Geometry: final body of the model. Coordinates: model frame, mm. A direction names the side the tool comes from. Coordinates: 2 decimals unless noted, no trailing zeros. Order: outer loops, then holes, each group sorted by start corner. A loop starts at its lowest first (then second) coordinate and runs counter-clockwise, first axis right, second up. Notation, with made-up numbers: (81, 46.25) -> (105, 46.25) arc R24 ccw to (105, 83.25) -> close; hole circle Ø9 at (89.5, 74). An arc over 180 degrees is marked (long way). Answer in a Markdown table with one row per item. Add a question column.
1) Section query A-A on y = 0. Return the cut outline in (x, z).
2) Section query C-C on y = 28. Return the cut outline in (x, z), then the cut area to 3 significant figures.
3) Pull-direction query (Y, two-part tool) for faces 1 (the face through (40, 50.8, -1)), 2 (the face through (40, -50.8, -1)), 3 (the face through (40, -1, 50.8)), 4 (the face through (3.736, -18.163, 49.858)); classes: +Y half, -Y half, draft (parallel to the pull), parting line (faces both ways), or undercut.
4) Section query B-B on x = 69. Return the cut outline in (y, z).
5) Contact query for flat-ended pins moving along their axis: P1, Ø10, axis at y = 39, z = -19.5, coming from the +X side; P2, Ø0.5, axis at x = 15, z = 50.5, coming from the -Y side; P3, Ø1.7, axis at y = 4, z = 50, coming from the -X side. Output: stop coordinate, or through.
6) Set-up query: faces 5 (the face through (3.736, 18.163, 49.858)), 6 (the face through (40.915, 47.827, -47.748)), 7 (the face through (0.95, 0.64, 48.68)). Return all of +Z, -Z, +X, -X, +Y, -Y with unobstructed straight access to the full face (end or side cutting, diameter ignored); none if empty.
7) Section query D-D on z = -5. Return the cut outline in (x, y).
8) Ray query, line 1 (Y direction, x = 37, z = -44.5); line 2 (Z direction, x = 39, y = -30); line 3 (X direction, y = -6.5, z = -31). Return the intervals inside material, ascending. Write a range as from..to.
```python
from build123d import *

# Parameters (mm, degrees)
F0_W          = 101.6
F0_H          = 101.6
F0_W_2        = 98.552
F0_H_2        = 98.552
F1_DEPTH      = 76.2
F2_W          = 101.6
F2_H          = 101.6
F3_DEPTH      = 1.524
F4_W          = 38.1
F4_H          = 38.1
F5_DEPTH      = 1.524
F6_R          = 5.08
F7_R          = 5.08
F10_T1_DEPTH  = 93.472
F10_T3_DEPTH  = 88.392
F10_T5_DEPTH  = 74.676
F10_T7_DEPTH  = 69.596
F10_S11_W     = 5.08
F10_S11_H     = 5.08
F10_T12_DEPTH = 5.08
F10_S17_W     = 5.08
F10_S17_H     = 5.08
F10_T18_DEPTH = 5.08
F10_T21_DEPTH = 91.44
F10_T23_DEPTH = 91.44
F10_T26_ANGLE = 90
F10_T28_ANGLE = 90
F10_T30_ANGLE = 90
F10_T32_ANGLE = 90


# Not quite as in the source:
# - a fillet or chamfer that OpenCascade refuses, or shapes differently, is made with other operations: its cross-section is extruded or revolved along the edge and cut away or added
# - a feature of the source that left no trace in its solid (it failed there, or was rolled back) is left out


with BuildPart() as f1:
    # F0 (on Right) → F1 (new body)
    with BuildSketch(Plane.YZ):
        Rectangle(F0_W, F0_H)
        Rectangle(F0_W_2, F0_H_2, mode=Mode.SUBTRACT)
    extrude(amount=F1_DEPTH)

    # F2 (on Right) → F3 (join)
    with BuildSketch(Plane.YZ):
        Rectangle(F2_W, F2_H)
    extrude(amount=F3_DEPTH)

    # F4 (on face) → F5 (cut)
    with BuildSketch(Plane.XY.offset(50.8)):
        with Locations((20.574, 0)):
            Rectangle(F4_W, F4_H)
    extrude(amount=-F5_DEPTH, mode=Mode.SUBTRACT)

    # F6
    f6_edges = [f1.edges().sort_by_distance(p)[0] for p in [
        (39.624, 19.05, 50.038),
        (39.624, -19.05, 50.038),
        (1.524, -19.05, 50.038),
        (1.524, 19.05, 50.038),
    ]]
    fillet(f6_edges, radius=F6_R)

    # F7
    f7_edges = [f1.edges().sort_by_distance(p)[0] for p in [
        (38.1, 50.8, 50.8),
        (38.1, -50.8, 50.8),
        (38.1, -50.8, -50.8),
        (38.1, 50.8, -50.8),
    ]]
    fillet(f7_edges, radius=F7_R)

    # F10: fillet of radius 5.08 on 15 edges, made by hand

    # F10_s2 → F10_t1 (join)
    with BuildSketch(Plane.XY.offset(-44.196)):
        with BuildLine():
            ThreePointArc((1.524, 44.196), (3.0118975516, 47.7881024484), (6.604, 49.276))
            Line((6.604, 49.276), (1.524, 49.276))
            Line((1.524, 49.276), (1.524, 44.196))
        make_face()
        with BuildLine():
            ThreePointArc((1.524, -44.196), (3.0118975516, -47.7881024484), (6.604, -49.276))
            Line((6.604, -49.276), (1.524, -49.276))
            Line((1.524, -49.276), (1.524, -44.196))
        make_face()
    extrude(amount=F10_T1_DEPTH)

    # F10_s4 → F10_t3 (join)
    with BuildSketch(Plane.XZ.offset(-44.196)):
        with BuildLine():
            ThreePointArc((1.524, -44.196), (3.0118975516, -47.7881024484), (6.604, -49.276))
            Line((6.604, -49.276), (1.524, -49.276))
            Line((1.524, -49.276), (1.524, -44.196))
        make_face()
    extrude(amount=F10_T3_DEPTH)

    # F10_s6 → F10_t5 (join)
    with BuildSketch(Plane.YZ.offset(1.524)):
        with BuildLine():
            ThreePointArc((-49.276, 44.196), (-47.7881024484, 47.7881024484), (-44.196, 49.276))
            Line((-44.196, 49.276), (-49.276, 49.276))
            Line((-49.276, 49.276), (-49.276, 44.196))
        make_face()
        with BuildLine():
            ThreePointArc((44.196, 49.276), (47.7881024484, 47.7881024484), (49.276, 44.196))
            Line((49.276, 44.196), (49.276, 49.276))
            Line((49.276, 49.276), (44.196, 49.276))
        make_face()
    extrude(amount=F10_T5_DEPTH)

    # F10_s8 → F10_t7 (join)
    with BuildSketch(Plane.YZ.offset(6.604)):
        with BuildLine():
            ThreePointArc((-49.276, -44.196), (-47.7881024484, -47.7881024484), (-44.196, -49.276))
            Line((-44.196, -49.276), (-49.276, -49.276))
            Line((-49.276, -49.276), (-49.276, -44.196))
        make_face()
        with BuildLine():
            ThreePointArc((49.276, -44.196), (47.7881024484, -47.7881024484), (44.196, -49.276))
            Line((44.196, -49.276), (49.276, -49.276))
            Line((49.276, -49.276), (49.276, -44.196))
        make_face()
    extrude(amount=F10_T7_DEPTH)


with BuildPart() as f10_tool10:
    # F10_s11 → F10_t12 (new body)
    with BuildSketch(Plane.XY.offset(-44.196)):
        with Locations((4.064, 46.736)):
            Rectangle(F10_S11_W, F10_S11_H)
    extrude(amount=-F10_T12_DEPTH)

    # F10_s13 → F10_t14 (revolve, cut)
    with BuildSketch(Plane(origin=(6.604, 44.196, -44.196), x_dir=(0.7071067812, -0.7071067812, 0), z_dir=(0.7071067812, 0.7071067812, 0))):
        with BuildLine():
            ThreePointArc((0, -5.08), (5.08, 0), (0, 5.08))
            Line((0, 5.08), (0, -5.08))
        make_face()
    revolve(axis=Axis((6.604, 44.196, -44.196), (0, 0, -1)), mode=Mode.SUBTRACT)


with BuildPart() as f1_1:
    add(f1.part)

    # F10_t9: union F10_tool10
    add(f10_tool10.part)


with BuildPart() as f10_tool16:
    # F10_s17 → F10_t18 (new body)
    with BuildSketch(Plane.XY.offset(-44.196)):
        with Locations((4.064, -46.736)):
            Rectangle(F10_S17_W, F10_S17_H)
    extrude(amount=-F10_T18_DEPTH)

    # F10_s19 → F10_t20 (revolve, cut)
    with BuildSketch(Plane(origin=(6.604, -44.196, -44.196), x_dir=(0.7071067812, 0.7071067812, 0), z_dir=(-0.7071067812, 0.7071067812, 0))):
        with BuildLine():
            ThreePointArc((0, -5.08), (5.08, 0), (0, 5.08))
            Line((0, 5.08), (0, -5.08))
        make_face()
    revolve(axis=Axis((6.604, -44.196, -44.196), (0, 0, -1)), mode=Mode.SUBTRACT)


with BuildPart() as f1_2:
    add(f1_1.part)

    # F10_t15: union F10_tool16
    add(f10_tool16.part)

    # F10_s22 → F10_t21 (cut)
    with BuildSketch(Plane.XZ.offset(-45.72)):
        with BuildLine():
            ThreePointArc((5.08, 50.8), (1.4878975516, 49.3121024484), (0, 45.72))
            Line((0, 45.72), (0, 50.8))
            Line((0, 50.8), (5.08, 50.8))
        make_face()
        with BuildLine():
            ThreePointArc((5.08, -50.8), (1.4878975516, -49.3121024484), (0, -45.72))
            Line((0, -45.72), (0, -50.8))
            Line((0, -50.8), (5.08, -50.8))
        make_face()
    extrude(amount=F10_T21_DEPTH, mode=Mode.SUBTRACT)

    # F10_s24 → F10_t23 (cut)
    with BuildSketch(Plane.XY.offset(-45.72)):
        with BuildLine():
            ThreePointArc((5.08, 50.8), (1.4878975516, 49.3121024484), (0, 45.72))
            Line((0, 45.72), (0, 50.8))
            Line((0, 50.8), (5.08, 50.8))
        make_face()
        with BuildLine():
            ThreePointArc((5.08, -50.8), (1.4878975516, -49.3121024484), (0, -45.72))
            Line((0, -45.72), (0, -50.8))
            Line((0, -50.8), (5.08, -50.8))
        make_face()
    extrude(amount=F10_T23_DEPTH, mode=Mode.SUBTRACT)

    # F10_s25 → F10_t26 (revolve, cut)
    with BuildSketch(Plane.XY.offset(-45.72)):
        with BuildLine():
            ThreePointArc((5.08, 50.8), (1.4878975516, 49.3121024484), (0, 45.72))
            Line((0, 45.72), (0, 50.8))
            Line((0, 50.8), (5.08, 50.8))
        make_face()
    revolve(axis=Axis((0, 45.72, -45.72), (-1, 0, 0)), revolution_arc=F10_T26_ANGLE, mode=Mode.SUBTRACT)

    # F10_s27 → F10_t28 (revolve, cut)
    with BuildSketch(Plane.XZ.offset(-45.72)):
        with BuildLine():
            ThreePointArc((5.08, 50.8), (1.4878975516, 49.3121024484), (0, 45.72))
            Line((0, 45.72), (0, 50.8))
            Line((0, 50.8), (5.08, 50.8))
        make_face()
    revolve(axis=Axis((0, 45.72, 45.72), (-1, 0, 0)), revolution_arc=F10_T28_ANGLE, mode=Mode.SUBTRACT)

    # F10_s29 → F10_t30 (revolve, cut)
    with BuildSketch(Plane.XY.offset(-45.72)):
        with BuildLine():
            ThreePointArc((5.08, -50.8), (1.4878975516, -49.3121024484), (0, -45.72))
            Line((0, -45.72), (0, -50.8))
            Line((0, -50.8), (5.08, -50.8))
        make_face()
    revolve(axis=Axis((0, -45.72, -45.72), (1, 0, 0)), revolution_arc=F10_T30_ANGLE, mode=Mode.SUBTRACT)

    # F10_s31 → F10_t32 (revolve, cut)
    with BuildSketch(Plane.XZ.offset(45.72)):
        with BuildLine():
            ThreePointArc((5.08, 50.8), (1.4878975516, 49.3121024484), (0, 45.72))
            Line((0, 45.72), (0, 50.8))
            Line((0, 50.8), (5.08, 50.8))
        make_face()
    revolve(axis=Axis((0, -45.72, 45.72), (1, 0, 0)), revolution_arc=F10_T32_ANGLE, mode=Mode.SUBTRACT)


solid = f1_2.part
```
Result:
| question | item | result |
|---|---|---|
| 1 | outline | (0, -45.72) arc R5.08 ccw to (5.08, -50.8) -> (76.2, -50.8) -> (76.2, -49.28) -> (6.6, -49.28) arc R5.08 cw to (1.52, -44.2) -> (1.52, 49.35) arc R5.08 ccw to (0, 45.72) -> close; (39.62, 49.28) -> (76.2, 49.28) -> (76.2, 50.8) -> (39.62, 50.8) -> close |
| 2 | outline | (0, -45.72) arc R5.08 ccw to (5.08, -50.8) -> (76.2, -50.8) -> (76.2, -49.28) -> (6.6, -49.28) arc R5.08 cw to (1.52, -44.2) -> (1.52, 49.28) -> (76.2, 49.28) -> (76.2, 50.8) -> (5.08, 50.8) arc R5.08 ccw to (0, 45.72) -> close |
| 2 | area | 377 mm2 |
| 3 | face 1 | +Y half |
| 3 | face 2 | -Y half |
| 3 | face 3 | draft |
| 3 | face 4 | undercut |
| 4 | outline | (-50.8, -45.72) arc R5.08 ccw to (-45.72, -50.8) -> (45.72, -50.8) arc R5.08 ccw to (50.8, -45.72) -> (50.8, 45.72) arc R5.08 ccw to (45.72, 50.8) -> (-45.72, 50.8) arc R5.08 ccw to (-50.8, 45.72) -> close; hole (-49.28, -44.2) arc R5.08 ccw to (-44.2, -49.28) -> (44.2, -49.28) arc R5.08 ccw to (49.28, -44.2) -> (49.28, 44.2) arc R5.08 ccw to (44.2, 49.28) -> (-44.2, 49.28) arc R5.08 ccw to (-49.28, 44.2) -> close |
| 5 | P1 | x = 1.52 |
| 5 | P2 | y = -48.02 |
| 5 | P3 | x = 1.33 |
| 6 | face 5 | +Z |
| 6 | face 6 | +X |
| 6 | face 7 | +Z, -X, +Y, -Y |
| 7 | outline | (0, -45.72) arc R5.08 ccw to (5.08, -50.8) -> (76.2, -50.8) -> (76.2, -49.28) -> (6.6, -49.28) arc R5.08 cw to (1.52, -44.2) -> (1.52, 44.2) arc R5.08 cw to (6.6, 49.28) -> (76.2, 49.28) -> (76.2, 50.8) -> (5.08, 50.8) arc R5.08 ccw to (0, 45.72) -> close |
| 8 | line 1 | -50.8..-49.27, 49.27..50.8 |
| 8 | line 2 | -50.8..-49.28, 49.28..50.8 |
| 8 | line 3 | 0..1.52 |
